from build123d import *

# Parameters (mm, degrees)
F3_DEPTH  = 2.5
F5_DEPTH  = 297.5
F8_DEPTH  = 600
F10_DEPTH = 297.5


with BuildPart() as f3:
    # F0 (on Top) → F3 (new body, symmetric)
    with BuildSketch(Plane.XY):
        Polygon((-300, 0), (0, 0), (300, 0), (300, 140), (-300, 140), align=None)
    extrude(amount=F3_DEPTH, both=True)

    # F4 (on offset) → F5 (join)
    with BuildSketch(Plane.YZ.offset(2.5)):
        Polygon((0, 2.5), (0, 0), (0, -2.5), (140, -2.5), (120, 2.5), align=None)
        with BuildLine():
            ThreePointArc((24, 22.0959179423), (7.3508893593, 17.9919333848), (0, 2.5))
            Line((0, 2.5), (120, 2.5))
            Line((120, 2.5), (24, 22.0959179423))
        make_face()
        Polygon((140, 2.5), (120, 2.5), (140, -2.5), align=None)
    extrude(amount=F5_DEPTH)

    # F7 (on offset) → F8 (cut)
    with BuildSketch(Plane(origin=(-300, 0, 0), x_dir=(0, -1, 0), z_dir=(-1, 0, 0))):
        Polygon((-140, -2.5), (-120, 2.5), (-140, 2.5), align=None)
    extrude(amount=-F8_DEPTH, mode=Mode.SUBTRACT)

    # F9 (on offset) → F10 (join)
    with BuildSketch(Plane.YZ.offset(-2.5)):
        with BuildLine():
            ThreePointArc((24, 22.0959179423), (7.3508893593, 17.9919333848), (0, 2.5))
            Line((0, 2.5), (120, 2.5))
            Line((120, 2.5), (24, 22.0959179423))
        make_face()
        Polygon((0, 2.5), (0, 0), (0, -2.5), (140, -2.5), (120, 2.5), align=None)
    extrude(amount=-F10_DEPTH)


solid = f3.part
Read the model definition and answer for the solid it produces. Units are mm, in the model's axes. A direction names the side the tool comes from. Coordinates: 2 decimals unless noted, no trailing zeros. Order: outer loops, then holes, each group sorted by start corner. A loop starts at its lowest first (then second) coordinate and runs counter-clockwise, first axis right, second up. Notation, with made-up numbers: (40, 0) -> (84, 0) arc R8 cw to (84, 14) -> close; hole circle Ø11 at (15, -23.75). An arc over 180 degrees is marked (long way). Answer as a JSON object with one key per item and string values.
1) A tool of negligible diameter and unlimited length cuts with its end or side. For faces 4 (the face through (2.5, 46, 10)), 5 (the face through (-4, 71, -2.5)), from which of +Z, -Z, +X, -X, +Y, -Y can it reach the whole face along a straight path? Write none if from no direction.
Model answer:
{"face 4": "+Z, +Y, -Y", "face 5": "-Z, +X, -X, +Y, -Y"}
2) A cutting plane is placed at A-A, the plane z = 8.25. Determine the outline of the cut face in (x, y), plus the area to 3 significant figures.
Model answer:
{"outline": "(-300, 0.84) -> (-2.5, 0.84) -> (-2.5, 91.83) -> (-300, 91.83) -> close; (2.5, 0.84) -> (300, 0.84) -> (300, 91.83) -> (2.5, 91.83) -> close", "area": "54,100 mm²"}
3) A cutting plane is placed at B-B, the plane x = -171. Determine the outline of the cut face in (y, z).
Model answer:
{"outline": "(0, -2.5) -> (140, -2.5) -> (120, 2.5) -> (24, 22.1) arc R20 ccw to (0, 2.5) -> close"}
4) A cutting plane is placed at C-C, the plane y = 45. Determine the outline of the cut face in (x, z).
Model answer:
{"outline": "(-300, -2.5) -> (300, -2.5) -> (300, 17.81) -> (2.5, 17.81) -> (2.5, 2.5) -> (-2.5, 2.5) -> (-2.5, 17.81) -> (-300, 17.81) -> close"}
5) A cutting plane is placed at D-D, the plane y = 11. Determine the outline of the cut face in (x, z).
Model answer:
{"outline": "(-300, -2.5) -> (300, -2.5) -> (300, 20.36) -> (2.5, 20.36) -> (2.5, 2.5) -> (-2.5, 2.5) -> (-2.5, 20.36) -> (-300, 20.36) -> close"}
6) The mould has two halves that part along X. Classify faces 1 (the face through (300, 53, 7)), 2 (the face through (-300, 53, 7)), 3 (the face through (-2.5, 46, 10)): released by +X, released by -X, zero draft, split by the parting line, or undercut.
Model answer:
{"face 1": "released by +X", "face 2": "released by -X", "face 3": "undercut"}
7) Consider line 1 along X through (y, z) = (29, 7); line 2 along Z through (x, y) = (-1.5, 47.5); line 3 along Z through (x, y) = (-270.5, 20.5). Determine where each line is inside the solid, lowest interval first. Write a range as from..to.
Model answer:
{"line 1": "x = -300..-2.5, 2.5..300", "line 2": "z = -2.5..2.5", "line 3": "z = -2.5..22.49"}
8) Each of these flat-tipped pins is pushed along its axis until it touches: pin 1 (5 mm diameter, centred on y = 80.5, z = 14.5, fed in from +X); pin 2 (2.5 mm diameter, centred on x = 1, y = 35.5, fed in from +Z). Where does it stop, or does it pass through?
Model answer:
{"pin 1": "passes through", "pin 2": "stops at z = 2.5"}
